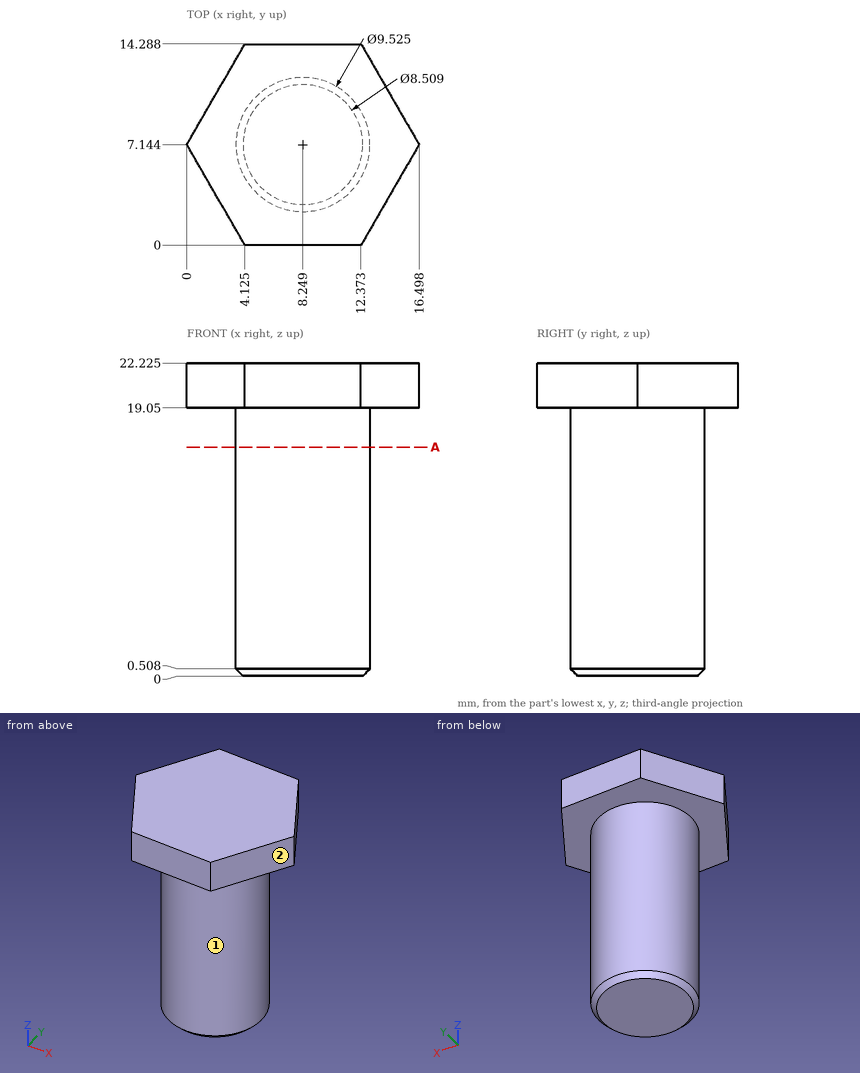
Print and shaded views of the part. All mm, measured from the part's lowest x, y and z. A direction names the side the tool comes from. Give positions to 0.01 mm unless a question says otherwise; leave off trailing zeros. Order: outer loops, then holes, each group sorted by start corner. A loop starts at its lowest first (then second) coordinate and runs counter-clockwise, first axis right, second up. Notation, with made-up numbers: (33, -34) - (84, -34) arc R26 ccw to (84, -9) - close; hole circle Ø9 at (62.5, 84.25). An arc over 180 degrees is marked (long way). One line per item, written item: value.
Item 1: Pin check, flat tips, straight feed: pin 1 Ø8 at (y, z) = (11.5, 12.5) entering from -X; pin 2 Ø6 at (x, z) = (2, 4) entering from -Y; pin 3 Ø6 at (y, z) = (3, 18.5) entering from +X. Stop position of each tip, or through.
Response values:
pin 1: x = 3.5
pin 2: y = 3.66
pin 3: x = 15.81
Item 2: Tool access for the marked faces 1 and 2: list every direction of +Z, -Z, +X, -X, +Y, -Y with a clear straight run to the whole face (end or side of a thin tool).
Response values:
face 1: -Z
face 2: +Z, -Z, +X, -Y
Item 3: Wall check: line 1 (Y direction, x = 8.25, z = 2); line 2 (X direction, y = 4, z = 16.75) (1 decimal); line 3 (X direction, y = 11.5, z = 17.75) (1 decimal). Give the ranges that are in metal, low to high.
Response values:
line 1: 2.38 to 11.91
line 2: 4.7 to 11.8
line 3: 6.3 to 10.2
Item 4: Slice it at A-A (z = 16.25). List the corners of the cut face in (x, y) (1 decimal).
Response values:
outline: circle Ø9.5 at (8.2, 7.1)
